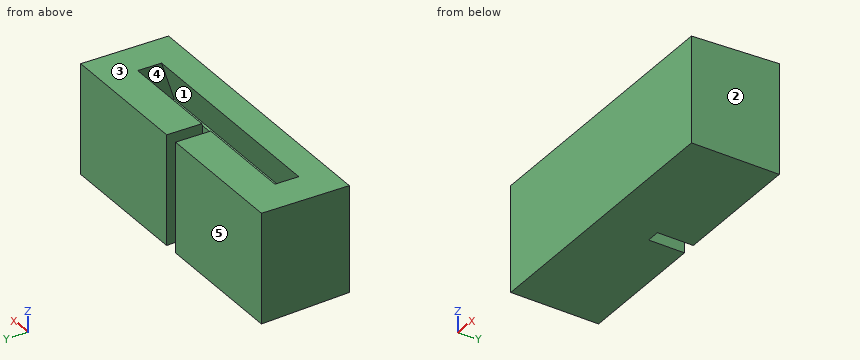
```python
from build123d import *

# Parameters (mm, degrees)
F0_W          = 108.712
F0_H          = 34.798
F1_DEPTH      = 43.688
F3_DEPTH      = 108.713
F4_W          = 5.334
F4_H          = 43.688
F5_DEPTH      = 14.224
F7_DEPTH      = 41.275
F7_DEPTH_BACK = 41.275


with BuildPart() as f1:
    # F0 (on Top) → F1 (new body)
    with BuildSketch(Plane.XY):
        with Locations((0, -6.154203)):
            Rectangle(F0_W, F0_H)
    extrude(amount=F1_DEPTH)

    # F2 (on face) → F3 (cut, through all)
    with BuildSketch(Plane.YZ.offset(54.356)):
        Polygon((-23.553203, 42.164), (11.244797, 43.688), (-23.553203, 43.688), align=None)
    extrude(amount=-F3_DEPTH, mode=Mode.SUBTRACT)

    # F4 (on face) → F5 (cut)
    with BuildSketch(Plane(origin=(0, 11.244797, 0), x_dir=(-1, 0, 0), z_dir=(0, 1, 0))):
        with Locations((0, 21.844)):
            Rectangle(F4_W, F4_H)
    extrude(amount=-F5_DEPTH, mode=Mode.SUBTRACT)

    # F6 (on Right) → F7 (cut, two sides)
    with BuildSketch(Plane.YZ) as f7_sk:
        Polygon((-8.7243, 23.997865), (3.653318, 63.273063), (-5.817524, 62.797693), (-17.203203, 26.67), align=None)
    extrude(amount=F7_DEPTH, mode=Mode.SUBTRACT)
    extrude(f7_sk.sketch, amount=-F7_DEPTH_BACK, mode=Mode.SUBTRACT)


solid = f1.part
```
Check sheet for the modelled part. Datum: model origin and axes. Units: mm. Face numbers are marked on the shaded views. A direction names the side the tool comes from. Round coordinates to 2 decimals unless told otherwise and drop trailing zeros. Write each loop counter-clockwise with the first axis right and the second up, starting at its lowest first coordinate (ties: lowest second). Pieces come first, ordered by that corner, then holes. Notation, with made-up numbers: (22, 50.5) -> (79, 50.5) arc R16 cw to (79, 63.5) -> close; hole circle Ø7 at (35, 89.25). An arc over 180 degrees is marked (long way). Put each result on its own line as item: value.
(1) Sectioned sample at C-C (x = 26.5). Enter the section's corners in (y, z), plus the area to 3 significant figures.
Values found:
outline: (-23.55, 0) -> (11.24, 0) -> (11.24, 43.69) -> (-2.71, 43.08) -> (-8.72, 24) -> (-17.2, 26.67) -> (-12.16, 42.66) -> (-23.55, 42.16) -> close
area: 1,330 mm^2
(2) Sectioned sample at D-D (y = -14). Enter the section's corners in (x, z) (1 decimal).
Values found:
outline: (-54.4, 0) -> (54.4, 0) -> (54.4, 42.6) -> (-54.4, 42.6) -> close; hole (-41.3, 25.7) -> (41.3, 25.7) -> (41.3, 36.8) -> (-41.3, 36.8) -> close
(3) Material ranges on line 1 (X direction, y = -2, z = 26); line 2 (Y direction, x = 3, z = 29); line 3 (Y direction, x = 4, z = 37), recorded low to high.
Values found:
line 1: x = -54.36 to -2.67, 2.67 to 54.36
line 2: y = -23.55 to -16.47, -7.15 to 11.24
line 3: y = -23.55 to -13.95, -4.63 to 11.24
(4) Go/stop test with flat-tipped pins: pin 1 Ø2.5 at (x, z) = (-1, 17.5) entering from +Y; pin 2 Ø2 at (x, y) = (41.5, 2) entering from +Z; pin 3 Ø1.5 at (x, y) = (3, -11) entering from +Z. Record where each tip stops, or that it passes through.
Values found:
pin 1: stops at y = -2.98
pin 2: stops at z = 43.33
pin 3: stops at z = 24.95
(5) Tool access check on the marked faces 1 and 2. Record the directions out of +Z, -Z, +X, -X, +Y, -Y that give a thin tool (end or side, any length) a straight path to the whole face; none if there is none.
Values found:
face 1: none
face 2: +Z, -Z, +X, +Y, -Y
(6) Sectioned sample at B-B (z = 9.5). Enter the section's corners in (x, y), plus the area to 3 significant figures.
Values found:
outline: (-54.36, -23.55) -> (54.36, -23.55) -> (54.36, 11.24) -> (2.67, 11.24) -> (2.67, -2.98) -> (-2.67, -2.98) -> (-2.67, 11.24) -> (-54.36, 11.24) -> close
area: 3,710 mm^2
(7) Sectioned sample at A-A (y = 3). Enter the section's corners in (x, z), plus the area to 3 significant figures.
Values found:
outline: (-54.36, 0) -> (-2.67, 0) -> (-2.67, 43.33) -> (-54.36, 43.33) -> close; (2.67, 0) -> (54.36, 0) -> (54.36, 43.33) -> (2.67, 43.33) -> close
area: 4,480 mm^2
(8) Mould release check, pull along Z, two halves, no side actions. Record for the marked faces 3, 4 and 5: released by +Z, released by -Z, zero draft, split by the parting line, or undercut.
Values found:
face 3: released by +Z
face 4: undercut
face 5: zero draft
